Here's the drawing with two shaded views (mm, measured from the low corner). I have some questions. Coordinates: 2 decimals unless noted, no trailing zeros. Loops run counter-clockwise (first coordinate to the right, second up) from the corner with the lowest first, then second, coordinate; pieces in that order, holes last.
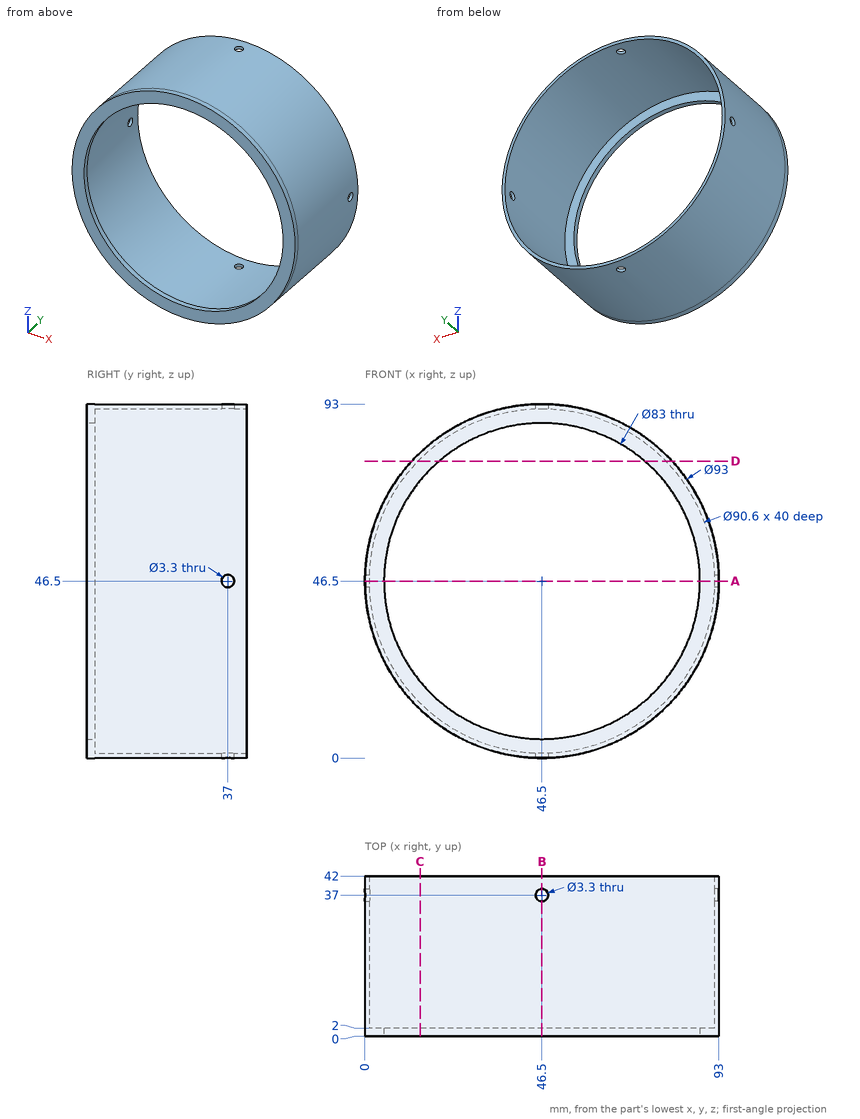
(1) I want a section at C-C on x = 14.5. Write out the boundary of the cut face in (y, z), then the cut area to 3 significant figures.
Check values:
outline: (0, 12.76) - (42, 12.76) - (42, 14.44) - (2, 14.44) - (2, 20.08) - (0, 20.08) - close; (0, 72.92) - (2, 72.92) - (2, 78.56) - (42, 78.56) - (42, 80.24) - (0, 80.24) - close
area: 163 mm2
(2) I'm going to push flat-ended pins straight in: pin 1 (5 mm diameter, centred on x = 9.5, y = 23.5, fed in from -Z); pin 2 (5 mm diameter, centred on y = 5, z = 17.5, fed in from +X); pin 3 (8 mm diameter, centred on y = 13, z = 13.5, fed in from +X). Where does each tip first touch, or does it pass through?
Check values:
pin 1: stops at z = 15.32
pin 2: stops at x = 84.71
pin 3: stops at x = 82.85
(3) I want a section at B-B on x = 46.5. Write out the boundary of the cut face in (y, z).
Check values:
outline: (0, 0) - (35.35, 0) - (35.35, 1.2) - (2, 1.2) - (2, 5) - (0, 5) - close; (0, 88) - (2, 88) - (2, 91.8) - (35.35, 91.8) - (35.35, 93) - (0, 93) - close; (38.65, 0) - (42, 0) - (42, 1.2) - (38.65, 1.2) - close; (38.65, 91.8) - (42, 91.8) - (42, 93) - (38.65, 93) - close
(4) I want a section at A-A on z = 46.5. Write out the boundary of the cut face in (x, y).
Check values:
outline: (0, 0) - (5, 0) - (5, 2) - (1.2, 2) - (1.2, 35.35) - (0, 35.35) - close; (0, 38.65) - (1.2, 38.65) - (1.2, 42) - (0, 42) - close; (88, 0) - (93, 0) - (93, 35.35) - (91.8, 35.35) - (91.8, 2) - (88, 2) - close; (91.8, 38.65) - (93, 38.65) - (93, 42) - (91.8, 42) - close
(5) If I drill on probe 1 along Y at (x, z) = (0.4, 46.5); probe 2 along X at (y, z) = (23.5, 46.5); probe 3 along X at (y, z) = (1, 46), over which ranges is the centre line in solid material (lowest first)?
Check values:
probe 1: y = 0 to 35.35, 38.65 to 42
probe 2: x = 0 to 1.2, 91.8 to 93
probe 3: x = 0 to 5, 88 to 93
(6) I want a section at D-D on z = 78. Write out the boundary of the cut face in (x, y), then the cut area to 3 significant figures.
Check values:
outline: (12.29, 0) - (19.48, 0) - (19.48, 2) - (13.94, 2) - (13.94, 42) - (12.29, 42) - close; (73.52, 0) - (80.71, 0) - (80.71, 42) - (79.06, 42) - (79.06, 2) - (73.52, 2) - close
area: 161 mm2
